```python
from build123d import *

# Parameters (mm, degrees)
SKETCH_1_W      = 19.8
SKETCH_1_H      = 10.2
SKETCH_1_R      = 1.25
EXTRUDE_1_DEPTH = 6.4


with BuildPart() as part:
    # 草图1 → 凸台-拉伸1 (new body)
    # profile 1 of 3: a face of its own
    with BuildSketch(Plane.XY):
        with Locations((4.8, 2.6)):
            Rectangle(SKETCH_1_W, SKETCH_1_H)
        with Locations((9.5, 0)):
            Circle(SKETCH_1_R, mode=Mode.SUBTRACT)
        Circle(SKETCH_1_R, mode=Mode.SUBTRACT)
    # profile 2 of 3: a face of its own
    with BuildSketch(Plane.XY):
        Polygon((-2.1, 8.7), (-2.1, 7.7), (-1.1, 7.7), (-1.1, 8.520009061), align=None)
    # profile 3 of 3: a face of its own
    with BuildSketch(Plane.XY):
        Polygon((-2.1, 8.7), (25.05212145, 14.356691969), (25.256075705, 13.377711549), (-1.1, 8.520009061), align=None)
    extrude(amount=EXTRUDE_1_DEPTH)


solid = part.part
```
CAD build for the part. Positions are in the model's coordinates, mm. A direction names the side the tool comes from. Coordinates: 2 decimals unless noted, no trailing zeros. Write each loop counter-clockwise with the first axis right and the second up, starting at its lowest first coordinate (ties: lowest second). Pieces come first, ordered by that corner, then holes.
(1) Cut at B-B, the plane x = 0. List the corners of the cut face in (y, z).
(2) Cut at C-C, the plane z = 2.25. List the corners of the cut face in (x, y), and give its area (3 significant figures).
(3) Flat gauge pins, fed straight in: pin 1 (0.9 mm diameter, centred on y = 8, z = 2.5, fed in from +X); pin 2 (1.9 mm diameter, centred on x = 8.5, z = 4, fed in from +Y); pin 3 (3 mm diameter, centred on x = 19.5, z = 5.5, fed in from +Y). Where does each tip first touch, or does it go through?
(4) 3-axis set-ups, long thin cutter, end or side, ignore diameter. For faces 5 (the face through (7, 4, 6.4)), 6 (the face through (-4, 7.7, 3)), 7 (the face through (7, 7.7, 3)): which of +Z, -Z, +X, -X, +Y, -Y reach the whole face in a straight line?
(5) Cut at D-D, the plane x = 14. List the corners of the cut face in (y, z).
(6) Drill centre lines: probe 1 along Y at (x, z) = (0, 4); probe 2 along Y at (x, z) = (9.5, 2.25); probe 3 along X at (y, z) = (7, 3). Where is each one in solid material? Low to high.
(7) Two-plate mould, pull along Y, no slides. Class faces 1 (the face through (5, -2.5, 3)), 2 (the face through (25.153, 13.874, 3.155)), 3 (the face through (12.263, 10.983, 3.155)), 4 (the face through (14.7, 3, 3)): +Y half, -Y half, draft (parallel to the pull), parting line (faces both ways), or undercut.
(8) Cut at A-A, the plane y = 0.75. List the corners of the cut face in (x, z), and give its area (3 significant figures).
Geometry says:
1. outline: (-2.5, 0) - (-1.25, 0) - (-1.25, 6.4) - (-2.5, 6.4) - close; (1.25, 0) - (7.7, 0) - (7.7, 6.4) - (1.25, 6.4) - close; (8.72, 0) - (9.14, 0) - (9.14, 6.4) - (8.72, 6.4) - close
2. outline: (-5.1, -2.5) - (14.7, -2.5) - (14.7, 7.7) - (-1.1, 7.7) - (-1.1, 8.52) - (25.26, 13.38) - (25.05, 14.36) - (-2.1, 8.7) - (-2.1, 7.7) - (-5.1, 7.7) - close; hole circle Ø2.5 at (0, 0); hole circle Ø2.5 at (9.5, 0)
2. area: 212 mm2
3. pin 1: stops at x = 14.7
3. pin 2: stops at y = 11.11
3. pin 3: stops at y = 13.51
4. face 5: +Z, +X, -X, +Y, -Y
4. face 6: +Z, -Z, -X, +Y
4. face 7: +Z, -Z, +X
5. outline: (-2.5, 0) - (7.7, 0) - (7.7, 6.4) - (-2.5, 6.4) - close; (11.3, 0) - (12.05, 0) - (12.05, 6.4) - (11.3, 6.4) - close
6. probe 1: y = -2.5 to -1.25, 1.25 to 7.7, 8.72 to 9.14
6. probe 2: y = -2.5 to -1.25, 1.25 to 7.7, 10.47 to 11.12
6. probe 3: x = -5.1 to 14.7
7. face 1: -Y half
7. face 2: +Y half
7. face 3: undercut
7. face 4: draft
8. outline: (-5.1, 0) - (-1, 0) - (-1, 6.4) - (-5.1, 6.4) - close; (1, 0) - (8.5, 0) - (8.5, 6.4) - (1, 6.4) - close; (10.5, 0) - (14.7, 0) - (14.7, 6.4) - (10.5, 6.4) - close
8. area: 101 mm2
